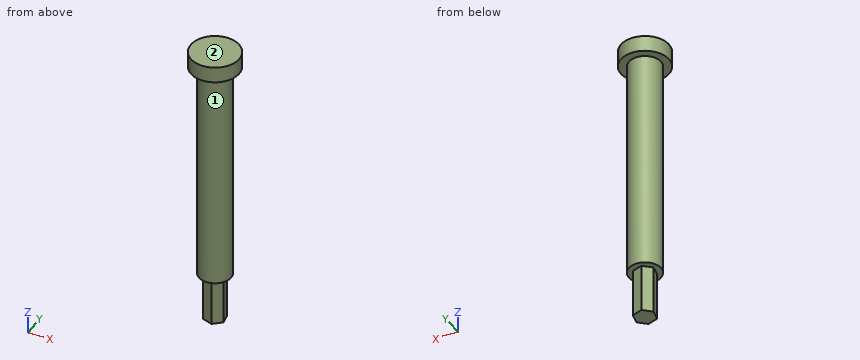
from build123d import *

# Parameters (mm, degrees)
BOSS_EXTRU_1_DEPTH = 15
ESQUISSE2_R        = 5
BOSS_EXTRU_2_DEPTH = 70
ESQUISSE3_R        = 7.5
BOSS_EXTRU_3_DEPTH = 5


with BuildPart() as part:
    # Esquisse1 → Boss.-Extru.1 (new body)
    with BuildSketch(Plane.XY):
        Polygon((-0.686649648, 3.395366293), (-3.283798289, 1.103027108), (-2.597148641, -2.292339185), (0.686649648, -3.395366293), (3.283798289, -1.103027108), (2.597148641, 2.292339185), align=None)
    extrude(amount=BOSS_EXTRU_1_DEPTH)

    # Esquisse2 → Boss.-Extru.2 (add)
    with BuildSketch(Plane.XY.offset(15)):
        Circle(ESQUISSE2_R)
    extrude(amount=BOSS_EXTRU_2_DEPTH)

    # Esquisse3 → Boss.-Extru.3 (add)
    with BuildSketch(Plane.XY.offset(85)):
        Circle(ESQUISSE3_R)
    extrude(amount=BOSS_EXTRU_3_DEPTH)


solid = part.part
Work out the finished part from the listing and answer in its coordinate system (mm). Face numbers are marked on the shaded views. A direction names the side the tool comes from. Give positions to 0.01 mm unless a question says otherwise; leave off trailing zeros. Order: outer loops, then holes, each group sorted by start corner. A loop starts at its lowest first (then second) coordinate and runs counter-clockwise, first axis right, second up. Notation, with made-up numbers: M 71.5,22.5 L 130.5,22.5 A29 ccw 130.5,49.5 Z; hole C 34.5,25 d3. An arc over 180 degrees is marked long. Return JSON: item names as keys, results as strings.
Q1. Find section C-C, the plane z = 40. Write down the section's boundary in (x, y), and give its area (3 significant figures).
Answer below:
{"outline": "C 0,0 d10", "area": "78.5 mm^2"}
Q2. Find section D-D, the plane y = 0. Write down the section's boundary in (x, z), and give its area (3 significant figures).
Answer below:
{"outline": "M -7.5,85 L -5,85 L -5,15 L -3.06,15 L -3.06,0 L 3.06,0 L 3.06,15 L 5,15 L 5,85 L 7.5,85 L 7.5,90 L -7.5,90 Z", "area": "867 mm^2"}
Q3. Each of these flat-tipped pins is pushed along its axis until it touches: pin 1 (8 mm diameter, centred on y = -1, z = 38.5, fed in from +X); pin 2 (8 mm diameter, centred on x = 5, z = 52.5, fed in from +Y); pin 3 (1 mm diameter, centred on y = -3, z = 67, fed in from +X); pin 4 (1.5 mm diameter, centred on y = -6, z = 20, fed in from +X). Where does it stop, or does it pass through?
Answer below:
{"pin 1": "stops at x = 5", "pin 2": "stops at y = 4.9", "pin 3": "stops at x = 4.33", "pin 4": "passes through"}
Q4. Find section A-A, the plane x = -6. Write down the section's boundary in (y, z).
Answer below:
{"outline": "M -4.5,85 L 4.5,85 L 4.5,90 L -4.5,90 Z"}
Q5. Find the intervals of material crossed by line 1 along Z through (x, y) = (-4.5, 3.5); line 2 along Z through (x, y) = (-1, -3); line 3 along Y through (x, z) = (-2.25, 77.5), in increasing order. Write a range as [from, to].
Answer below:
{"line 1": "z = [85, 90]", "line 2": "z = [15, 90]", "line 3": "y = [-4.47, 4.47]"}
Q6. Which of the six approach directions +Z, -Z, +X, -X, +Y, -Y give full straight-line access (tool end or side, diameter ignored) to the marked faces 1 and 2?
Answer below:
{"face 1": "-Z", "face 2": "+Z, +X, -X, +Y, -Y"}
